from build123d import *

# Parameters (mm, degrees)
BOSS_EXTRUDE1_DEPTH = 2
BOSS_EXTRUDE2_DEPTH = 200
SKETCH3_R           = 7.5
CUT_EXTRUDE1_DEPTH  = 200


with BuildPart() as part:
    # Sketch1 → Boss-Extrude1 (new body)
    with BuildSketch(Plane.XY):
        Polygon((10.574219011, 19.4635226), (22.256543634, 19.4635226), (35.076132829, 0), (20, -20), (0, -20), align=None)
    boss_extrude1 = extrude(amount=BOSS_EXTRUDE1_DEPTH)

    # Sketch2 → Boss-Extrude2 (add)
    with BuildSketch(Plane.XY.offset(2)):
        Polygon((10.574219011, 19.4635226), (12.574219011, 19.4635226), (2, -20), (0, -20), align=None)
    extrude(amount=-BOSS_EXTRUDE2_DEPTH)

    # Mirror1: Boss-Extrude1 across plane
    add(boss_extrude1.mirror(Plane.XY.offset(-98)))

    # Sketch3 → Cut-Extrude1 (cut)
    with BuildSketch(Plane(origin=(6.866025404, -1.839745962, 0), x_dir=(0, 0, -1), z_dir=(0.9659258262890692, -0.25881904510251774, 0))):
        with Locations(Location((58, 1.626944036, 0), (0, 0, 90))):
            Circle(SKETCH3_R)
        with Locations(Location((33, 1.626944036, 0), (0, 0, 90))):
            Circle(SKETCH3_R)
        with Locations(Location((163, 1.626944036, 0), (0, 0, 270))):
            Circle(SKETCH3_R)
        with Locations(Location((138, 1.626944036, 0), (0, 0, 270))):
            Circle(SKETCH3_R)
    extrude(amount=-CUT_EXTRUDE1_DEPTH, mode=Mode.SUBTRACT)


solid = part.part
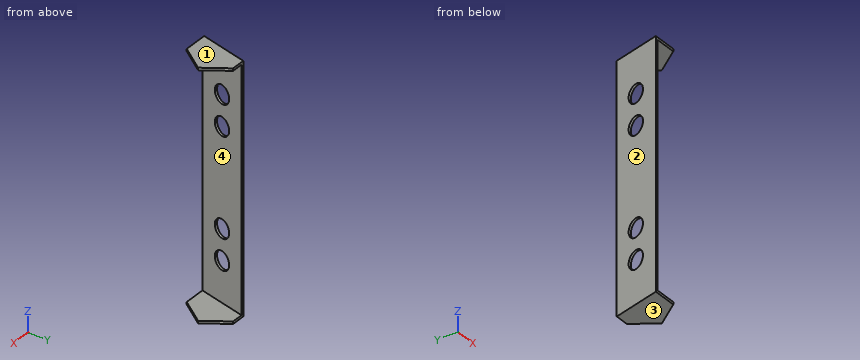
For this review, take the finished solid that the model builds, in its own axes (mm). Face numbers are marked on the shaded views. Give positions to 0.01 mm unless a question says otherwise; leave off trailing zeros. Loops run counter-clockwise (first coordinate to the right, second up) from the corner with the lowest first, then second, coordinate; pieces in that order, holes last.
Item 1: Take a section at A-A, the plane z = -134. State the section outline as (x, y) points.
Item 2: Insertion check: pin 1 (4 mm diameter, centred on y = 15, z = -175.5, fed in from +X); pin 2 (6 mm diameter, centred on y = 3, z = -174, fed in from -X); pin 3 (3 mm diameter, centred on y = 3.5, z = -159, fed in from +X); pin 4 (1 mm diameter, centred on y = 8, z = -177.5, fed in from -X). Each pin has a flat end and moves straight along its axis. Give the tip position at first contact, or say it passes through.
Item 3: Take a section at C-C, the plane y = 9.5. State the section outline as (x, z) points, and give its area (3 significant figures).
Item 4: Take a section at B-B, the plane x = 28. State the section outline as (y, z) points.
Item 5: Take a section at D-D, the plane y = 2. Give the number of separate pieces and of enclosed holes in the cut face, and give its area (3 significant figures).
Item 6: Draft analysis for pull direction Z (two halves, no side actions). For the marked faces 1, 2, 3 and 4, state which applies: +Z half, -Z half, draft (parallel to the pull), parting line (faces both ways), or undercut.
Item 7: For line 1 along Z through (x, y) = (25.5, 4.5); line 2 along X through (y, z) = (-13, -55); line 3 along X through (y, z) = (-5, -150.5), list the stretches that pass through material, from the lowest coordinate up.
Calculated:
1. outline: (0, -20) - (2, -20) - (5.65, -6.4) - (3.78, -5.9) - close; (7.06, 6.36) - (8.93, 5.86) - (12.57, 19.46) - (10.57, 19.46) - close
2. pin 1: stops at x = 11.91
2. pin 2: stops at x = 5.36
2. pin 3: passes through
2. pin 4: stops at x = 7.37
3. outline: (7.9, -198) - (28.82, -198) - (28.82, -196) - (9.9, -196) - (9.9, 0) - (28.82, 0) - (28.82, 2) - (7.9, 2) - close
3. area: 476 mm2
4. outline: (-9.39, -198) - (10.74, -198) - (10.74, -196) - (-9.39, -196) - close; (-9.39, 0) - (10.74, 0) - (10.74, 2) - (-9.39, 2) - close
5. separate pieces: 5
5. enclosed holes: 0
5. area: 388 mm2
6. face 1: +Z half
6. face 2: draft
6. face 3: -Z half
6. face 4: undercut
7. line 1: z = -198 to -196, 0 to 2
7. line 2: x = 1.88 to 3.88
7. line 3: x = 4.02 to 6.02
